Input: part model. Units: mm. Frame: model coordinates. A direction names the side the tool comes from. Give positions to 0.01 mm unless a question says otherwise; leave off trailing zeros. Loops run counter-clockwise (first coordinate to the right, second up) from the corner with the lowest first, then second, coordinate; pieces in that order, holes last. Notation, with made-up numbers: M -31.5,-21.75 L -27.5,-21.75 A15 cw -27.5,-12.75 Z; hole C 59.5,80.25 d8. An arc over 180 degrees is marked long. Return JSON: item names as keys, results as strings. Group by question number.
```python
from build123d import *

# Parameters (mm, degrees)
SKETCH1_W           = 20
SKETCH1_H           = 16.3
BOSS_EXTRUDE1_DEPTH = 260
CUT_EXTRUDE1_DEPTH  = 521
CHAMFER1_SIZE       = 1
FILLET1_R           = 1
CUT_EXTRUDE2_DEPTH  = 521
SKETCH4_R           = 4.75
SKETCH4_R_2         = 3
CUT_EXTRUDE3_DEPTH  = 8.5
SKETCH4_2_R         = 3
CUT_EXTRUDE4_DEPTH  = 17.3
LPATTERN1_COUNT     = 9
LPATTERN1_PITCH     = 60


with BuildPart() as part:
    # Sketch1 → Boss-Extrude1 (new body, symmetric)
    with BuildSketch(Plane.XY):
        with Locations((0, 8.15)):
            Rectangle(SKETCH1_W, SKETCH1_H)
    extrude(amount=BOSS_EXTRUDE1_DEPTH, both=True)

    # Sketch2 → Cut-Extrude1 (cut, through all)
    with BuildSketch(Plane.XY.offset(260)):
        Polygon((-10, 14.3), (-10, 7.3), (-7.666666667, 9.633333333), (-7.666666667, 11.966666667), align=None)
        Polygon((7.666666667, 11.966666667), (10, 14.3), (10, 7.3), (7.666666667, 9.633333333), align=None)
    extrude(amount=-CUT_EXTRUDE1_DEPTH, mode=Mode.SUBTRACT)

    # Chamfer1
    chamfer1_edges = [part.edges().sort_by_distance(p)[0] for p in [
        (-10, 16.3, 0),
        (10, 16.3, 0),
        (10, 0, 0),
        (-10, 0, 0),
    ]]
    chamfer(chamfer1_edges, length=CHAMFER1_SIZE)

    # Fillet1
    fillet1_edges = [part.edges().sort_by_distance(p)[0] for p in [
        (-7.666666667, 11.966666667, 0),
        (-7.666666667, 9.633333333, 0),
        (7.666666667, 9.633333333, 0),
        (7.666666667, 11.966666667, 0),
    ]]
    fillet(fillet1_edges, radius=FILLET1_R)

    # Sketch3 → Cut-Extrude2 (cut, through all)
    with BuildSketch(Plane.XY.offset(260)):
        Polygon((-6, 0), (-5, 1), (5, 1), (6, 0), align=None)
    extrude(amount=-CUT_EXTRUDE2_DEPTH, mode=Mode.SUBTRACT)

    # Sketch4 → Cut-Extrude3 (cut)
    with BuildSketch(Plane(origin=(0, 16.3, 0), x_dir=(1, 0, 0), z_dir=(0, 1, 0))):
        with Locations((0, -240)):
            Circle(SKETCH4_R)
        with Locations((0, -240)):
            Circle(SKETCH4_R_2, mode=Mode.SUBTRACT)
    cut_extrude3 = extrude(amount=-CUT_EXTRUDE3_DEPTH, mode=Mode.SUBTRACT)

    # Sketch4_2 → Cut-Extrude4 (cut, through all)
    with BuildSketch(Plane(origin=(0, 16.3, 0), x_dir=(1, 0, 0), z_dir=(0, 1, 0))):
        with Locations((0, -240)):
            Circle(SKETCH4_2_R)
    cut_extrude4 = extrude(amount=-CUT_EXTRUDE4_DEPTH, mode=Mode.SUBTRACT)

    # LPattern1: Cut-Extrude3, Cut-Extrude4 ×9
    with Locations(*[(0, 0, -i * LPATTERN1_PITCH) for i in range(1, LPATTERN1_COUNT)]):
        add(cut_extrude3, mode=Mode.SUBTRACT)
        add(cut_extrude4, mode=Mode.SUBTRACT)


solid = part.part
```
Item 1: Reachability of faces 3 (the face through (-1.03, 12.11, -175.363)), 4 (the face through (0, 1, 4)), 5 (the face through (-4, 16.3, 4)) from +Z, -Z, +X, -X, +Y, -Y: full face, straight path, thin tool, end or side. Return the list, or none.
Item 2: Pull-direction query (X, two-part tool) for faces 1 (the face through (0, 8, 260)), 2 (the face through (-1.03, 12.11, 124.637)); classes: pulls with the +X half, pulls with the -X half, needs draft (parallel to the pull), parting line crosses it, or undercut.
Item 3: Section A-A, the plane z = -150. Return loops of the section in (x, y).
Item 4: First-contact query: pin 1 Ø3 at (x, z) = (-1.5, -242) entering from +Y; pin 2 Ø5.5 at (x, z) = (0, -180) entering from -Y; pin 3 Ø8.5 at (x, z) = (0, 60) entering from -Y; pin 4 Ø10.5 at (x, z) = (-2, 240) entering from +Y. Flat tips, straight axial feed; report the tip coordinate or a pass-through.
Item 5: Material intervals for line 1 (X direction, y = 11.5, z = 120); line 2 (X direction, y = 3.25, z = 240); line 3 (Y direction, x = 3, z = 237.5), sorted ascending. Write a range as from..to.
Answer below:
{
 "1": {"face 3": "+Y", "face 4": "+Z, -Z, -Y", "face 5": "+Z, -Z, +X, -X, +Y"},
 "2": {"face 1": "needs draft", "face 2": "undercut"},
 "3": {"outline": "M -10,1 L -9,0 L -6,0 L -5,1 L 5,1 L 6,0 L 9,0 L 10,1 L 10,7.3 L 7.96,9.34 A1 cw 7.67,10.05 L 7.67,11.55 A1 cw 7.96,12.26 L 10,14.3 L 10,15.3 L 9,16.3 L -9,16.3 L -10,15.3 L -10,14.3 L -7.96,12.26 A1 cw -7.67,11.55 L -7.67,10.05 A1 cw -7.96,9.34 L -10,7.3 Z"},
 "4": {"pin 1": "y = 7.8", "pin 2": "through", "pin 3": "y = 1", "pin 4": "y = 16.3"},
 "5": {"line 1": "-7.67..-4.75, 4.75..7.67", "line 2": "-10..-3, 3..10", "line 3": "1..7.8"}
}
